Part model, mm, in its own coordinate system. A direction names the side the tool comes from. Give positions to 0.01 mm unless a question says otherwise; leave off trailing zeros. Loops run counter-clockwise (first coordinate to the right, second up) from the corner with the lowest first, then second, coordinate; pieces in that order, holes last. Notation, with made-up numbers: M -8.75,49.5 L 15.25,49.5 A6 cw 15.25,60.5 Z; hole C 56,26.25 d1. An arc over 180 degrees is marked long. Answer in a Markdown table with one row per item.
Autodesk Inventor part; units mm, degrees
ref_plane "Work Plane1" through (0, 0, 10) normal (0, 0, -1) x (-1, 0, 0)
ref_plane "YZ Plane" through (0, 0, 0) normal (1, 0, 0) x (0, 1, 0)
ref_plane "XZ Plane" through (0, 0, 0) normal (0, 1, 0) x (-1, 0, 0)
sketch "Sketch1" plane through (0, 0, 0) normal (0, 0, 1) x (1, 0, 0)
  circle A0 centre (0, 0) radius 5
  dimension "d0" = 10
extrude "Extrusion1" add sketch "Sketch1" along normal blind 10
sketch "Sketch2" plane through (0, 0, 10) normal (0, 0, 1) x (1, 0, 0)
  circle A0 centre (0, 0) radius 5
  circle A1 centre (0, 0) radius 4.445
  dimension "d3" = 8.89
extrude "Extrusion2" add sketch "Sketch2" along normal blind 12.7
sketch "Sketch3" plane through (0, 0, 10) normal (0, 0, 1) x (1, 0, 0)
  circle A0 centre (0, 0) radius 3.175
  dimension "d8" = 6.35
extrude "Extrusion3" cut sketch "Sketch3" against normal blind 12.7
thread "Thread2"
ref_plane "Work Plane1" through (0, 0, 10) normal (0, 0, -1) x (-1, 0, 0)
sketch "Sketch4" plane through (0, 0, 10) normal (0, 0, -1) x (-1, 0, 0)
  circle A0 centre (0, 0) radius 6
  circle A1 centre (0, 0) radius 5
  dimension "d14" = 12
extrude "Extrusion4" add sketch "Sketch4" along normal blind 1
thread "Thread3"
properties part number "Pedal Connector Right"
(1) Which spindle directions (+Z, -Z, +X, -X, +Y, -Y) get a long thin tool onto all of the face, cutting with end or side? Do faces 1 (the face through (-0.69, -3.1, 5.07)), 2 (the face through (-0.96, 4.34, 16.26)), 3 (the face through (4, 4, 9)). Say none if no direction does.
Recorded:
| item | result |
|---|---|
| face 1 | +Z, -Z |
| face 2 | +Z |
| face 3 | -Z |
(2) Saw through at C-C (z = 7.25). Write the cut outline in (x, y) (3 decimals).
Recorded:
| item | result |
|---|---|
| outline | C 0,0 d10; hole C 0,0 d6.35 |
(3) Saw through at A-A (y = 0). Write the cut outline in (x, z) (3 decimals), plus the area to 3 significant figures.
Recorded:
| item | result |
|---|---|
| outline | M -6,9 L -5,9 L -5,0 L -3.175,0 L -3.175,10 L -4.445,10 L -4.445,22.7 L -5,22.7 L -5,10 L -6,10 Z; M 3.175,0 L 5,0 L 5,9 L 6,9 L 6,10 L 5,10 L 5,22.7 L 4.445,22.7 L 4.445,10 L 3.175,10 Z |
| area | 52.6 mm^2 |
(4) Saw through at D-D (z = 20). Write the cut outline in (x, y) (3 decimals).
Recorded:
| item | result |
|---|---|
| outline | C 0,0 d10; hole C 0,0 d8.89 |
(5) Pull direction X, two halves, no side cores. Call faces 4 (the face through (5.994, -0.264, 9.507)), 5 (the face through (2, -3, 10)), 6 (the face through (4, 4, 10)): +X half, -X half, draft (parallel to the pull), parting line (faces both ways), or undercut.
Recorded:
| item | result |
|---|---|
| face 4 | parting line |
| face 5 | undercut |
| face 6 | draft |
(6) Pin check, flat tips, straight feed: pin 1 Ø5 at (x, z) = (3, 13.5) entering from +Y; pin 2 Ø6 at (y, z) = (3.5, 10.5) entering from -X; pin 3 Ø5 at (x, z) = (-4.5, 16.5) entering from -Y; pin 4 Ø5.5 at (x, y) = (0, 0) entering from -Z. Stop position of each tip, or through.
Recorded:
| item | result |
|---|---|
| pin 1 | stops at y = 4.97 |
| pin 2 | stops at x = -5.98 |
| pin 3 | stops at y = -4.58 |
| pin 4 | passes through |
(7) Drill centre lines: line 1 along Y through (x, z) = (0, 7.5) (3 decimals); line 2 along Y through (x, z) = (0, 19.5) (3 decimals); line 3 along Z through (x, y) = (3.5, 4). Where is each one in solid material? Low to high.
Recorded:
| item | result |
|---|---|
| line 1 | y = -5 to -3.175, 3.175 to 5 |
| line 2 | y = -5 to -4.445, 4.445 to 5 |
| line 3 | z = 9 to 10 |
